from build123d import *

# Parameters (mm, degrees)
SKETCH2_R             = 80.5
SKETCH2_R_2           = 5
BOSS_EXTRUDE1_DEPTH   = 1.5
BOSS_EXTRUDE3_DEPTH   = 5
BOSS_EXTRUDE3_DRAFT   = 30
BOSS_EXTRUDE3_2_DEPTH = 5
BOSS_EXTRUDE3_2_DRAFT = 30
BOSS_EXTRUDE4_DEPTH   = 7.5
SKETCH8_R             = 2
CUT_EXTRUDE1_DEPTH    = 3


# Read off the part's stored shape, not the designer's step: Boss-Extrude3
with BuildPart() as part:
    # Sketch2 → Boss-Extrude1 (new body)
    with BuildSketch(Plane(origin=(0, 0, 0), x_dir=(1, 0, 0), z_dir=(0, 1, 0))):
        with Locations(Location((0, 0, 0), (0, 0, 270))):
            Circle(SKETCH2_R)
        with Locations(Location((0, 0, 0), (0, 0, 270))):
            Circle(SKETCH2_R_2, mode=Mode.SUBTRACT)
    extrude(amount=BOSS_EXTRUDE1_DEPTH)


with BuildPart() as boss_extrude3_tool:
    # Boss-Extrude3 outline → Boss-Extrude3 (with draft: the straight prism first)
    with BuildSketch(Plane(origin=(0, 6.5, 0), x_dir=(1, 0, 0), z_dir=(0, 1, 0))):
        with BuildLine():
            Line((-7.598356857, 2.113248654), (-77.584473619, 2.113248654))
            ThreePointArc((-77.584473619, 2.113248654), (-77.613248654, 0), (-77.584473619, -2.113248654))
            Line((-77.584473619, -2.113248654), (-7.598356857, -2.113248654))
            ThreePointArc((-7.598356857, -2.113248654), (-7.886751346, 0), (-7.598356857, 2.113248654))
        make_face()
    extrude(amount=-BOSS_EXTRUDE3_DEPTH)
    # Boss-Extrude3: the draft: its side faces are tilted about the plane it starts from
    boss_extrude3_sides = [boss_extrude3_tool.faces().sort_by_distance(p)[0] for p in [
        (-42.591415238, 4, -2.113248654),
        (-77.613248654, 4, 0),
        (-42.591415238, 4, 2.113248654),
        (-7.886751346, 4, 0),
    ]]
    draft(boss_extrude3_sides, Plane(origin=(0, 6.5, 0), x_dir=(1, 0, 0), z_dir=(0, 1, 0)), BOSS_EXTRUDE3_DRAFT)


with BuildPart() as part_1:
    add(part.part)

    # Boss-Extrude3: add boss_extrude3_tool
    add(boss_extrude3_tool.part)


with BuildPart() as boss_extrude3_2_tool:
    # Boss-Extrude3 2 outline → Boss-Extrude3 2 (with draft: the straight prism first)
    with BuildSketch(Plane(origin=(0, 6.5, 0), x_dir=(1, 0, 0), z_dir=(0, 1, 0))):
        with BuildLine():
            Line((77.584473619, 2.113248654), (7.598356857, 2.113248654))
            ThreePointArc((7.598356857, 2.113248654), (7.886751346, 0), (7.598356857, -2.113248654))
            Line((7.598356857, -2.113248654), (77.584473619, -2.113248654))
            ThreePointArc((77.584473619, -2.113248654), (77.613248654, 0), (77.584473619, 2.113248654))
        make_face()
    extrude(amount=-BOSS_EXTRUDE3_2_DEPTH)
    # Boss-Extrude3 2: the draft: its side faces are tilted about the plane it starts from
    boss_extrude3_2_sides = [boss_extrude3_2_tool.faces().sort_by_distance(p)[0] for p in [
        (42.591415238, 4, 2.113248654),
        (77.613248654, 4, 0),
        (42.591415238, 4, -2.113248654),
        (7.886751346, 4, 0),
    ]]
    draft(boss_extrude3_2_sides, Plane(origin=(0, 6.5, 0), x_dir=(1, 0, 0), z_dir=(0, 1, 0)), BOSS_EXTRUDE3_2_DRAFT)


with BuildPart() as part_2:
    add(part_1.part)

    # Boss-Extrude3 2: add boss_extrude3_2_tool
    add(boss_extrude3_2_tool.part)

    # Sketch6 → Revolve1 (revolve)
    with BuildSketch(Plane.XY, mode=Mode.PRIVATE) as revolve1_sk:
        Polygon((-80.5, 0), (-82, 0), (-82, 14.2), (-75, 14.2), (-75, 12.7), (-80.5, 12.7), align=None)
    revolve(revolve1_sk.sketch.rotate(Axis((0, 13, 0), (0, -1, 0)), 270), axis=Axis((0, 13, 0), (0, -1, 0)))

    # Sketch7 → Boss-Extrude4 (add)
    with BuildSketch(Plane.XZ):
        with BuildLine():
            Line((10.405859981, 10), (14.903696288, 10))
            ThreePointArc((14.903696288, 10), (16.317909851, 9.414213562), (16.903696288, 8))
            Line((16.903696288, 8), (16.903696288, -8))
            ThreePointArc((16.903696288, -8), (16.317909851, -9.414213562), (14.903696288, -10))
            Line((14.903696288, -10), (10.405859981, -10))
            Line((10.405859981, -10), (10.405859981, 10))
        make_face()
        with BuildLine():
            Line((-30.594140019, -10), (-35.091976326, -10))
            ThreePointArc((-35.091976326, -10), (-36.506189888, -9.414213562), (-37.091976326, -8))
            Line((-37.091976326, -8), (-37.091976326, 8))
            ThreePointArc((-37.091976326, 8), (-36.506189888, 9.414213562), (-35.091976326, 10))
            Line((-35.091976326, 10), (-30.594140019, 10))
            Line((-30.594140019, 10), (-30.594140019, -10))
        make_face()
    extrude(amount=BOSS_EXTRUDE4_DEPTH)

    # Sketch8 → Cut-Extrude1 (cut)
    with BuildSketch(Plane.XZ.offset(7.5)):
        with Locations(Location((13.905859981, -5, 0), (0, 0, 270))):
            Circle(SKETCH8_R)
        with Locations(Location((13.905859981, 5, 0), (0, 0, 270))):
            Circle(SKETCH8_R)
        with Locations(Location((-34.094140019, -5, 0), (0, 0, 270))):
            Circle(SKETCH8_R)
        with Locations(Location((-34.094140019, 5, 0), (0, 0, 270))):
            Circle(SKETCH8_R)
    extrude(amount=-CUT_EXTRUDE1_DEPTH, mode=Mode.SUBTRACT)


solid = part_2.part
CAD build for the part. Positions are in the model's coordinates, mm. A direction names the side the tool comes from. Coordinates: 2 decimals unless noted, no trailing zeros. Write each loop counter-clockwise with the first axis right and the second up, starting at its lowest first coordinate (ties: lowest second). Pieces come first, ordered by that corner, then holes. Notation, with made-up numbers: (44, 69) - (97, 69) arc R27 cw to (97, 98) - close; hole circle Ø5 at (26.25, -28.5). An arc over 180 degrees is marked (long way). Use a Markdown table: item, result. Add a question column.
Item 1: Band-saw the part on C-C, the plane y = 9.25. Give the cut face in (x, z).
Item 2: Drill centre lines: L1, parallel to X at y = -6.7, z = -5; L2, parallel to X at y = 6, z = 0; L3, parallel to Y at x = 1.5, z = 42. Where is each one in solid material? Low to high. Write a range as from..to.
Item 3: Band-saw the part on D-D, the plane z = 29.5. Give the cut face in (x, y), and give its area (3 significant figures).
Item 4: Mould opens along Z. For faces 1 (the face through (10.406, -4, 0)), 2 (the face through (13, -4, 10)), 3 (the face through (14, -4.5, -5)) say: pulls with the +Z half, pulls with the -Z half, needs draft (parallel to the pull), parting line crosses it, or undercut.
Item 5: Flat gauge pins, fed straight in: pin 1 (10 mm diameter, centred on y = -3, z = -49.5, fed in from +X); pin 2 (8 mm diameter, centred on x = 29, y = -1.5, fed in from -Z); pin 3 (12 mm diameter, centred on y = 7, z = 40.5, fed in from -X). Where does each tip first touch, or does it go through?
Item 6: Band-saw the part on A-A, the plane z = 0. Give the cut face in (x, y), and give its area (3 significant figures).
Item 7: 3-axis set-ups, long thin cutter, end or side, ignore diameter. For faces 4 (the face through (-5.82, 2.92, 0.13)), 5 (the face through (15.89, -6.02, 5.26)), 6 (the face through (-36, 12.7, 66)), 7 (the face through (16.904, -4, 0)), 8 (the face through (-30.594, -4, 0)): which of +Z, -Z, +X, -X, +Y, -Y reach the whole face in a straight line?
Item 8: Band-saw the part on B-B, the plane x = 22. Give the cut face in (y, z).
Numbers:
| question | item | result |
|---|---|---|
| 1 | outline | circle Ø164 at (0, 0); hole circle Ø161 at (0, 0) |
| 2 | L1 | -37.09..-36.09, -32.09..-30.59, 10.41..11.91, 15.91..16.9 |
| 2 | L2 | -82..-80.5, -77.9..-7.6, 7.6..77.9, 80.5..82 |
| 2 | L3 | 0..1.5 |
| 3 | outline | (-76.51, 0) - (76.51, 0) - (76.51, 14.2) - (68.95, 14.2) - (68.95, 12.7) - (74.9, 12.7) - (74.9, 1.5) - (-74.9, 1.5) - (-74.9, 12.7) - (-68.95, 12.7) - (-68.95, 14.2) - (-76.51, 14.2) - close |
| 3 | area | 288 mm2 |
| 4 | face 1 | needs draft |
| 4 | face 2 | pulls with the +Z half |
| 4 | face 3 | undercut |
| 5 | pin 1 | x = 68.22 |
| 5 | pin 2 | z = -78 |
| 5 | pin 3 | x = -74.39 |
| 6 | outline | (-82, 0) - (-37.09, 0) - (-37.09, -7.5) - (-30.59, -7.5) - (-30.59, 0) - (-5, 0) - (-5, 1.5) - (-7.89, 6.5) - (-77.61, 6.5) - (-80.5, 1.5) - (-80.5, 12.7) - (-75, 12.7) - (-75, 14.2) - (-82, 14.2) - close; (5, 0) - (10.41, 0) - (10.41, -7.5) - (16.9, -7.5) - (16.9, 0) - (82, 0) - (82, 14.2) - (75, 14.2) - (75, 12.7) - (80.5, 12.7) - (80.5, 1.5) - (77.61, 6.5) - (7.89, 6.5) - (5, 1.5) - close |
| 6 | area | 1,110 mm2 |
| 7 | face 4 | +Y |
| 7 | face 5 | -Y |
| 7 | face 6 | none |
| 7 | face 7 | +Z, -Z, +X, -Y |
| 7 | face 8 | +Z, -Z, -Y |
| 8 | outline | (0, -78.99) - (14.2, -78.99) - (14.2, -71.7) - (12.7, -71.7) - (12.7, -77.44) - (1.5, -77.44) - (1.5, -5) - (6.5, -2.11) - (6.5, 2.11) - (1.5, 5) - (1.5, 77.44) - (12.7, 77.44) - (12.7, 71.7) - (14.2, 71.7) - (14.2, 78.99) - (0, 78.99) - close |
